from build123d import *

# Parameters (mm, degrees)
SKETCH1_W           = 75
SKETCH1_H           = 70
BOSS_EXTRUDE1_DEPTH = 5
SKETCH2_R           = 1.5
CUT_EXTRUDE1_DEPTH  = 59.699989832
CUT_EXTRUDE3_DEPTH  = 2.5


with BuildPart() as part:
    # Sketch1 → Boss-Extrude1 (new body)
    with BuildSketch(Plane(origin=(0, 0, 0), x_dir=(1, 0, 0), z_dir=(0, 1, 0))):
        with Locations((0, 9.8825)):
            Rectangle(SKETCH1_W, SKETCH1_H)
        with BuildLine():
            Line((-25.410018342, -2.5), (-8.306962441, -2.5))
            ThreePointArc((-8.306962441, -2.5), (0, -8.675), (8.306962441, -2.5))
            Line((8.306962441, -2.5), (25.410018342, -2.5))
            ThreePointArc((25.410018342, -2.5), (27.552103918, -1.600349825), (28.409437718, 0.559020409))
            ThreePointArc((28.409437718, 0.559020409), (0, 28.414937186), (-28.409437718, 0.559020409))
            ThreePointArc((-28.409437718, 0.559020409), (-27.552103918, -1.600349825), (-25.410018342, -2.5))
        make_face(mode=Mode.SUBTRACT)
    extrude(amount=BOSS_EXTRUDE1_DEPTH)

    # Sketch2 → Cut-Extrude1 (cut, through all)
    with BuildSketch(Plane(origin=(0, 5, 0), x_dir=(1, 0, 0), z_dir=(0, 1, 0))):
        with Locations(Location((-30, 38.3825, 0), (0, 0, 270))):
            Circle(SKETCH2_R)
        with Locations(Location((-30, -18.6175, 0), (0, 0, 270))):
            Circle(SKETCH2_R)
        with Locations(Location((0, -18.6175, 0), (0, 0, 270))):
            Circle(SKETCH2_R)
        with Locations(Location((30, -18.6175, 0), (0, 0, 270))):
            Circle(SKETCH2_R)
        with Locations(Location((30, 38.3825, 0), (0, 0, 270))):
            Circle(SKETCH2_R)
        with Locations(Location((0, 38.3825, 0), (0, 0, 270))):
            Circle(SKETCH2_R)
    extrude(amount=-CUT_EXTRUDE1_DEPTH, mode=Mode.SUBTRACT)

    # Sketch3 → Cut-Extrude3 (cut)
    with BuildSketch(Plane.XZ):
        with BuildLine():
            Line((25.410018342, 7.5), (11.434842587, 7.5))
            ThreePointArc((11.434842587, 7.5), (0, 13.675), (-11.434842587, 7.5))
            Line((-11.434842587, 7.5), (-25.410018342, 7.5))
            ThreePointArc((-25.410018342, 7.5), (-31.122246544, 5.100932866), (-33.408470011, -0.657387759))
            ThreePointArc((-33.408470011, -0.657387759), (0, -33.414937186), (33.408470011, -0.657387759))
            ThreePointArc((33.408470011, -0.657387759), (31.122246544, 5.100932866), (25.410018342, 7.5))
        make_face()
    extrude(amount=-CUT_EXTRUDE3_DEPTH, mode=Mode.SUBTRACT)


solid = part.part
Can you work these out from the model? Positions are in its coordinate system, mm. A direction names the side the tool comes from. Give positions to 0.01 mm unless a question says otherwise; leave off trailing zeros. Loops run counter-clockwise (first coordinate to the right, second up) from the corner with the lowest first, then second, coordinate; pieces in that order, holes last. Notation, with made-up numbers: M 17.25,49 L 60.25,49 A20 cw 60.25,86 Z; hole C 28,54 d11. An arc over 180 degrees is marked long. One line per item, written item: value. Start each with the question number.
1) If we section it at C-C, the plane z = -14.5: Write out the boundary of the cut face in (x, y).
2) If we section it at A-A, the plane y = 1.2: Give the number of separate pieces and of enclosed holes in the cut face, and give its area (3 significant figures).
3) If I drill on line 1 (Z direction, x = 29, y = 2.05); line 2 (Y direction, x = -7, z = 10.5); line 3 (X direction, y = 4.3, z = -1), over which ranges is the centre line in solid material (lowest first)? Write a range as [from, to].
4) If we section it at D-D, the plane z = 18.5: Write out the boundary of the cut face in (x, y), and give its area (3 significant figures).
5) Thinking about a two-plate mould opening in Z: for faces 4 (the face through (-27.575, 3.732, 1.576)), 5 (the face through (-1, 0, -34)), 6 (the face through (-1, 2, -44.882)), which applies, +Z half, -Z half, draft (parallel to the pull), parting line (faces both ways), or undercut?
6) If we section it at B-B, the plane x = 0: Write out the boundary of the cut face in (y, z) (1 decimal), and give its area (3 significant figures).
7) On a 3-axis mill with a long thin cutter (end or side, diameter ignored), from which of +Z, -Z, +X, -X, +Y, -Y can I reach the whole of each face in a straight line? I mean faces 1 (the face through (8, 5, 5)), 2 (the face through (-0.155, 3.732, 8.674)), 3 (the face through (0.19, 1.232, 13.674)). Say none if no direction works.
Completed:
1. outline: M -37.5,0 L -30.1,0 L -30.1,2.5 L -24.44,2.5 L -24.44,5 L -37.5,5 Z; M 24.44,2.5 L 30.1,2.5 L 30.1,0 L 37.5,0 L 37.5,5 L 24.44,5 Z
2. separate pieces: 1
2. enclosed holes: 7
2. area: 2,880 mm^2
3. line 1: z = [-44.88, -39.5], [-37.26, -16.6], [6.65, 17.5], [19.74, 25.12]
3. line 2: y = [2.5, 5]
3. line 3: x = [-37.5, -28.4], [28.4, 37.5]
4. outline: M -37.5,0 L -31.5,0 L -31.5,5 L -37.5,5 Z; M -28.5,0 L -1.5,0 L -1.5,5 L -28.5,5 Z; M 1.5,0 L 28.5,0 L 28.5,5 L 1.5,5 Z; M 31.5,0 L 37.5,0 L 37.5,5 L 31.5,5 Z
4. area: 330 mm^2
5. face 4: undercut
5. face 5: draft
5. face 6: -Z half
6. outline: M 0,-44.9 L 5,-44.9 L 5,-39.9 L 0,-39.9 Z; M 0,-36.9 L 5,-36.9 L 5,-28.4 L 2.5,-28.4 L 2.5,-33.4 L 0,-33.4 Z; M 0,13.7 L 2.5,13.7 L 2.5,8.7 L 5,8.7 L 5,17.1 L 0,17.1 Z; M 0,20.1 L 5,20.1 L 5,25.1 L 0,25.1 Z
6. area: 110 mm^2
7. face 1: +Z, -Z, +X, -X, +Y
7. face 2: +Y, -Y
7. face 3: -Y
